Autodesk Inventor part; units mm, degrees
ref_plane "YZ Plane" through (0, 0, 0) normal (1, 0, 0) x (0, 1, 0)
ref_plane "XZ Plane" through (0, 0, 0) normal (0, 1, 0) x (-1, 0, 0)
ref_plane "XY Plane" through (0, 0, 0) normal (0, 0, 1) x (1, 0, 0)
sketch "Sketch1" plane through (0, 0, 0) normal (0, 1, 0) x (-1, 0, 0)
  line L0 (0, 0) -> (20.32, 0)
  line L1 (20.32, 0) -> (20.32, -27.94)
  line L2 (20.32, -27.94) -> (0, -27.94)
  line L3 (0, -27.94) -> (0, 0)
  dimension "d0" = 20.32
  dimension "d1" = 27.94
extrude "Extrusion1" add sketch "Sketch1" along normal blind 12.7
sketch "Sketch2" plane through (-20.32, 0, 0) normal (0, 0, 1) x (1, 0, 0)
  line L0 (2.54, 2.54) -> (17.78, 2.54)
  line L1 (17.78, 2.54) -> (17.78, 10.16)
  line L2 (17.78, 10.16) -> (2.54, 10.16)
  line L3 (2.54, 10.16) -> (2.54, 2.54)
  point P0 (0, 0)
  dimension "d6" = 15.24
  dimension "d7" = 7.62
extrude "Extrusion2" cut sketch "Sketch2" against normal blind 22.86
sketch "Sketch3" plane through (0, 0, -27.94) normal (0, 0, -1) x (-1, 0, 0)
  line L0 (0, 0) -> (0, 12.7)
  line L1 (0, 0) -> (20.32, 0)
  line L2 (0, 12.7) -> (20.32, 12.7)
  line L3 (20.32, 12.7) -> (20.32, 0)
  line L4 (20.32, 0) -> (0, 0)
  line L5 (0, 0) -> (0, 12.7)
extrude "Extrusion3" cut sketch "Sketch3" against normal blind 2.54
sketch "Sketch4" plane through (0, 0, 0) normal (0, -1, 0) x (1, 0, 0)
  line L0 (-8.89, 0) -> (-11.43, 0)
  line L1 (-11.43, 0) -> (-11.43, -25.4)
  line L2 (-11.43, -25.4) -> (-8.89, -25.4)
  line L3 (-8.89, -25.4) -> (-8.89, 0)
  line L4 (-20.32, 0) -> (-20.32, -25.4)
  line L5 (0, -25.4) -> (0, 0)
  dimension "d12" = 8.89
  dimension "d32" = 8.89
sketch "Sketch5" plane through (0, 0, -25.4) normal (0, 0, -1) x (-1, 0, 0)
  line L0 (0, 0) -> (20.32, 0)
  line L1 (10.16, 0) -> (10.16, 6.35)
  circle A0 centre (10.16, 6.35) radius 1.27
  dimension "d14" = 6.35
  dimension "d15" = 2.54
extrude "Extrusion4" cut sketch "Sketch5" against normal blind 2.54
extrude "Extrusion5" cut sketch "Sketch4" against normal blind 6.35
sketch "Sketch8" plane through (0, 12.7, 0) normal (0, 1, 0) x (1, 0, 0)
  line L0 (0, 25.4) -> (0, 0)
  line L1 (-20.32, 0) -> (-20.32, 25.4)
  line L2 (0, 0) -> (-20.32, 0)
  line L3 (-20.32, 0) -> (-20.32, 12.7)
  line L4 (-20.32, 12.7) -> (0, 12.7)
  line L5 (0, 12.7) -> (0, 0)
extrude "Extrusion8" add sketch "Sketch8" along normal blind 2.54
sketch "Sketch9" plane through (-17.78, 10.16, 0) normal (0, 0, 1) x (1, 0, 0)
  arc A0 (8.89, -3.81) -> (6.35, -3.81) centre (7.62, -3.81) ccw
  line L0 (7.62, -3.81) -> (7.62, 7.62)
  point P0 (17.78, -10.16)
  dimension "d36" = 11.43
sketch "Sketch10" plane through (0, 15.24, 0) normal (0, 1, 0) x (1, 0, 0)
  line L0 (-11.43, 0) -> (-20.32, 0)
  line L1 (-20.32, 0) -> (0, 0)
  line L2 (0, 0) -> (0, 12.7)
  line L3 (0, 12.7) -> (-20.32, 12.7)
  line L4 (-20.32, 12.7) -> (-20.32, 0)
extrude "Extrusion9" cut sketch "Sketch10" against normal blind 1.27
sketch "Sketch11" plane through (0, 13.97, 0) normal (0, 1, 0) x (1, 0, 0)
  point P0 (0, 0)
sketch "Sketch12" plane through (0, 13.97, 0) normal (0, 1, 0) x (1, 0, 0)
  line L0 (-17.78, 0) -> (-2.54, 0)
  line L1 (-10.16, 0) -> (-10.16, 12.7099)
  line L2 (-10.16, 0) -> (-16.51, 0)
  line L3 (-11.43, 0) -> (-20.32, 0)
  line L4 (-10.16, 0) -> (-3.81, 0)
  line L5 (-3.81, 0) -> (0, 0)
  line L6 (0, 0) -> (0, 12.7099)
  line L7 (0, 12.7099) -> (-3.81, 12.7099)
  line L8 (-3.81, 12.7099) -> (-3.81, 0)
  line L9 (-20.32, 0) -> (-20.32, 12.7)
  line L10 (-16.51, 0) -> (-20.32, 0)
  line L11 (-20.32, 0) -> (-20.32, 12.7)
  line L12 (-20.32, 12.7) -> (-16.51, 12.7)
  line L13 (-16.51, 12.7) -> (-16.51, 0)
  dimension "d39" = 6.35
  dimension "d40" = 6.35
extrude "Extrusion10" add sketch "Sketch12" along normal blind 7.62
sketch "Sketch13" plane through (-17.78, 10.16, 0) normal (0, 0, 1) x (1, 0, 0)
  line L0 (17.78, 3.81) -> (17.78, 11.43)
  line L1 (1.27, 3.81) -> (13.97, 3.81)
  line L2 (17.78, 11.43) -> (13.97, 11.43)
  line L3 (13.97, 11.43) -> (13.97, 3.81)
  line L4 (13.97, 3.81) -> (17.78, 3.81)
  line L5 (17.78, 3.81) -> (17.78, 11.43)
  line L6 (1.27, 11.43) -> (-2.54, 11.43)
  line L7 (-2.54, 2.54) -> (-2.54, 11.43)
  line L8 (1.27, 11.43) -> (-2.54, 11.43)
  line L9 (-2.54, 11.43) -> (-2.54, 3.81)
  line L10 (-2.54, 3.81) -> (1.27, 3.81)
  line L11 (1.27, 3.81) -> (1.27, 11.43)
  point P0 (17.78, -10.16)
extrude "Extrusion11" add sketch "Sketch13" along normal blind 27.94
sketch "Sketch14" plane through (0, 0, 0) normal (1, 0, 0) x (0, 0, -1)
  line L0 (-27.94, 13.97) -> (-27.94, 21.59)
  line L1 (12.7, 21.59) -> (-27.94, 21.59)
  line L2 (-27.94, 13.97) -> (-22.86, 13.97)
  line L3 (-22.86, 13.97) -> (-22.86, 21.59)
  line L4 (-22.86, 21.59) -> (-27.94, 21.59)
  line L5 (-27.94, 21.59) -> (-27.94, 13.97)
  point P0 (0, 0)
  dimension "d45" = 5.08
sketch "Sketch15" plane through (0, 21.59, 0) normal (0, 1, 0) x (1, 0, 0)
  point P0 (0, 0)
extrude "Extrusion12" add sketch "Sketch14" along normal blind 2.54
sketch "Sketch16" plane through (-20.32, 0, -25.4) normal (-1, 0, 0) x (0, 0, 1)
  line L0 (48.26, 21.59) -> (53.34, 21.59)
  line L1 (53.34, 13.97) -> (48.26, 13.97)
  line L2 (53.34, 21.59) -> (48.26, 21.59)
  line L3 (48.26, 21.59) -> (48.26, 13.97)
  line L4 (48.26, 13.97) -> (53.34, 13.97)
  line L5 (53.34, 13.97) -> (53.34, 21.59)
  point P0 (25.4, 0)
extrude "Extrusion13" add sketch "Sketch16" along normal blind 2.54
chamfer "Chamfer3" distance 5.08 angle 45 1 edges at (-22.86, 17.78, 27.94)
chamfer "Chamfer4" distance 5.08 angle 45 1 edges at (2.54, 17.78, 27.94)
sketch "Sketch17" plane through (-20.32, 0, -25.4) normal (-1, 0, 0) x (0, 0, 1)
  line L0 (12.7, 12.7) -> (12.7, 21.59)
  line L1 (25.4, 13.97) -> (48.26, 13.97)
  line L2 (12.7, 21.59) -> (48.26, 21.59)
  line L3 (48.26, 21.59) -> (48.26, 13.97)
  line L4 (48.26, 13.97) -> (12.7, 13.97)
  line L5 (12.7, 13.97) -> (12.7, 21.59)
  point P0 (25.4, 0)
extrude "Extrusion14" cut sketch "Sketch17" against normal blind 1.27
sketch "Sketch18" plane through (0, 0, 0) normal (1, 0, 0) x (0, 0, -1)
  line L0 (12.7099, 13.97) -> (12.7099, 21.59)
  line L1 (0, 13.97) -> (-22.86, 13.97)
  line L2 (12.7099, 21.59) -> (-22.86, 21.59)
  line L3 (-22.86, 21.59) -> (-22.86, 13.97)
  line L4 (-22.86, 13.97) -> (12.7099, 13.97)
  line L5 (12.7099, 13.97) -> (12.7099, 21.59)
  point P0 (0, 0)
extrude "Extrusion15" cut sketch "Sketch18" against normal blind 1.27
properties part number "Small USB Cover"
Verification items for the finished model (mm, model axes). A direction names the side the tool comes from. Give positions to 0.01 mm unless a question says otherwise; leave off trailing zeros. Order: outer loops, then holes, each group sorted by start corner. A loop starts at its lowest first (then second) coordinate and runs counter-clockwise, first axis right, second up. Notation, with made-up numbers: M -22.75,4 L 15.25,4 A33 cw 15.25,36 Z; hole C 74.5,57 d7. An arc over 180 degrees is marked long. Return JSON: item names as keys, results as strings. Group by question number.
1) Section check A-A on z = 4. Record the cut outline in (x, y).
2) Section check C-C on x = -10.16. Record the cut outline in (y, z), and give its area (3 significant figures).
3) Scan lines: line 1 (X direction, y = 1.5, z = -11); line 2 (X direction, y = 15.5, z = 8.5); line 3 (Y direction, x = -7, z = -12). Record each from-to range of solid material in increasing order.
4) Mould release check, pull along X, two halves, no side actions. Record for faces 1 (the face through (-18, 21.59, 7)), 2 (the face through (-20.36, 17.83, 25.36)), 3 (the face through (-10, 10.16, -11)), 4 (the face through (-10.19, 7.62, -24.15)): pulls with the +X half, pulls with the -X half, needs draft (parallel to the pull), parting line crosses it, or undercut.
5) Go/stop test with flat-tipped pins: pin 1 Ø1 at (y, z) = (7, -7) entering from +X; pin 2 Ø11 at (y, z) = (10, -15) entering from -X; pin 3 Ø8.5 at (y, z) = (16, 16.5) entering from -X. Record where each tip stops, or that it passes through.
6) Access from +Z, -Z, +X, -X, +Y, -Y to the whole of each face (thin tool, end or side, straight path). Record for faces 5 (the face through (-2, 13.97, 14)), 6 (the face through (-19.05, 18, 5)), 7 (the face through (-1, 13.97, -6)), 8 (the face through (1, 18, 22.86)), 9 (the face through (-2.54, 6, -11)).
7) Section check D-D on z = -8. Record the cut outline in (x, y).
Answer block:
{
 "1": {"outline": "M -19.05,13.97 L -16.51,13.97 L -16.51,21.59 L -19.05,21.59 Z; M -3.81,13.97 L -1.27,13.97 L -1.27,21.59 L -3.81,21.59 Z"},
 "2": {"outline": "M 7.62,-25.4 L 12.7,-25.4 L 12.7,-12.7 L 13.97,-12.7 L 13.97,0 L 10.16,0 L 10.16,-22.86 L 7.62,-22.86 Z", "area": "87.1 mm^2"},
 "3": {"line 1": "x = -20.32 to -11.43, -8.89 to 0", "line 2": "x = -19.05 to -16.51, -3.81 to -1.27", "line 3": "y = 0 to 2.54, 10.16 to 13.97"},
 "4": {"face 1": "needs draft", "face 2": "pulls with the -X half", "face 3": "undercut", "face 4": "undercut"},
 "5": {"pin 1": "stops at x = 0", "pin 2": "stops at x = -20.32", "pin 3": "stops at x = -19.05"},
 "6": {"face 5": "+Z, +X, -X, -Y", "face 6": "-Z, -X, +Y", "face 7": "-Z, +X, +Y", "face 8": "-Z, +X, +Y, -Y", "face 9": "+Z"},
 "7": {"outline": "M -20.32,0 L -11.43,0 L -11.43,2.54 L -17.78,2.54 L -17.78,10.16 L -2.54,10.16 L -2.54,2.54 L -8.89,2.54 L -8.89,0 L 0,0 L 0,13.97 L -1.27,13.97 L -1.27,21.59 L -3.81,21.59 L -3.81,13.97 L -16.51,13.97 L -16.51,21.59 L -19.05,21.59 L -19.05,13.97 L -20.32,13.97 Z"}
}
